Model file for the job. Use its own axes, mm. A direction names the side the tool comes from. Round coordinates to 2 decimals unless told otherwise and drop trailing zeros. Order: outer loops, then holes, each group sorted by start corner. A loop starts at its lowest first (then second) coordinate and runs counter-clockwise, first axis right, second up. Notation, with made-up numbers: (74.5, -23) - (83.5, -23) arc R20 cw to (83.5, -9) - close; hole circle Ø2 at (81.25, 38). An arc over 180 degrees is marked (long way). Answer as CSV lines item,"result". Start each with the question number.
1. Band-saw the part on D-D on z = -4. List the corners of the cut face in (x, y).
2. 3-axis set-ups, long thin cutter, end or side, ignore diameter. For faces 1 (the face through (2, -12, -3)), 2 (the face through (-2, 7, 0)), 3 (the face through (19, 28, 0)): which of +Z, -Z, +X, -X, +Y, -Y reach the whole face in a straight line?
3. Pin check, flat tips, straight feed: pin 1 Ø4 at (x, z) = (2, 1.5) entering from -Y; pin 2 Ø2 at (x, z) = (1, 6) entering from -Y; pin 3 Ø1.5 at (x, z) = (-2, -2.5) entering from +Y; pin 4 Ø1.5 at (x, y) = (2, -13) entering from +Z. Stop position of each tip, or through.
4. Band-saw the part on B-B on y = 24.5. List the corners of the cut face in (x, z).
5. Band-saw the part on C-C on x = 0.75. List the corners of the cut face in (y, z).
6. Band-saw the part on A-A on z = 0. List the corners of the cut face in (x, y), then the cut area to 4 significant figures.
7. Wall check: line 1 along Z through (x, y) = (15.5, 25); line 2 along X through (y, z) = (28, 0.25); line 3 along Y through (x, z) = (2.15, 0). Give the ranges that are in metal, low to high. Write a range as [from, to].
8. Pull direction X, two halves, no side cores. Call faces 4 (the face through (2.46, -4.88, 1.08)), 5 (the face through (19, 8, -14)), 6 (the face through (13, 28, -3)): released by +X, released by -X, zero draft, split by the parting line, or undercut.
```python
from build123d import *

# Parameters (mm, degrees)
SKETCH_1_R          = 5
EXTRUDE_1_DEPTH     = 5
EXTRUDE_2_DEPTH     = 21
FILLET_1_R          = 5
SKETCH_3_W          = 30
SKETCH_3_H          = 27
EXTRUDE_3_DEPTH     = 5
CUT_EXTRUDE_1_DEPTH = 50.037074512


with BuildPart() as part:
    # Sketch 1 → Extrude 1 (new body)
    # profile 1 of 5: a face of its own
    with BuildSketch(Plane(origin=(0, 0, 0), x_dir=(0, 0, -1), z_dir=(1, 0, 0))):
        with BuildLine():
            Line((-15, 30), (15, 30))
            ThreePointArc((15, 30), (0, 45), (-15, 30))
        make_face()
    # profile 2 of 5: a face of its own
    with BuildSketch(Plane(origin=(0, 0, 0), x_dir=(0, 0, -1), z_dir=(1, 0, 0))):
        with BuildLine():
            Line((-15, 45), (-15, 30))
            ThreePointArc((-15, 30), (-10.606601718, 40.606601718), (0, 45))
            Line((0, 45), (-15, 45))
        make_face()
    # profile 3 of 5: a face of its own
    with BuildSketch(Plane(origin=(0, 0, 0), x_dir=(0, 0, -1), z_dir=(1, 0, 0))):
        with BuildLine():
            ThreePointArc((0, 45), (10.606601718, 40.606601718), (15, 30))
            Line((15, 30), (15, 45))
            Line((15, 45), (0, 45))
        make_face()
    # profile 4 of 5: a face of its own
    with BuildSketch(Plane(origin=(0, 0, 0), x_dir=(0, 0, -1), z_dir=(1, 0, 0))):
        with BuildLine():
            Line((-15, 7), (-15, 0))
            ThreePointArc((-15, 0), (-11.618950039, -9.486832981), (-3, -14.696938457))
            Line((-3, -14.696938457), (-3, -8.5))
            Line((-3, -8.5), (3, -8.5))
            Line((3, -8.5), (3, -14.696938457))
            ThreePointArc((3, -14.696938457), (11.618950039, -9.486832981), (15, 0))
            Line((15, 0), (15, 7))
            Line((15, 7), (12, 7))
            Line((12, 7), (12, 27))
            Line((12, 27), (-12, 27))
            Line((-12, 27), (-12, 7))
            Line((-12, 7), (-15, 7))
        make_face()
        Circle(SKETCH_1_R, mode=Mode.SUBTRACT)
    # profile 5 of 5: a face of its own
    with BuildSketch(Plane(origin=(0, 0, 0), x_dir=(0, 0, -1), z_dir=(1, 0, 0))):
        Polygon((-15, 30), (-15, 7), (-12, 7), (-12, 27), (12, 27), (12, 7), (15, 7), (15, 30), align=None)
    extrude(amount=EXTRUDE_1_DEPTH)

    # Sketch 1_4 → Extrude 2 (add)
    with BuildSketch(Plane(origin=(0, 0, 0), x_dir=(0, 0, -1), z_dir=(1, 0, 0))):
        Polygon((-15, 30), (-15, 7), (-12, 7), (-12, 27), (12, 27), (12, 7), (15, 7), (15, 30), align=None)
    extrude(amount=EXTRUDE_2_DEPTH)

    # Fillet 1
    fillet_1_edges = [part.edges().sort_by_distance(p)[0] for p in [
        (21, 7, -13.5),
        (21, 7, 13.5),
    ]]
    fillet(fillet_1_edges, radius=FILLET_1_R)

    # Sketch 3 → Extrude 3 (add)
    with BuildSketch(Plane.ZY):
        with Locations((0, 20.5)):
            Rectangle(SKETCH_3_W, SKETCH_3_H)
    extrude(amount=EXTRUDE_3_DEPTH)

    # Sketch 4 → Cut-Extrude 1 (cut, through all)
    with BuildSketch(Plane.XZ.offset(-27)):
        with BuildLine():
            Line((10, 3), (16, 3))
            ThreePointArc((16, 3), (19, 0), (16, -3))
            Line((16, -3), (10, -3))
            ThreePointArc((10, -3), (7, 0), (10, 3))
        make_face()
    extrude(amount=-CUT_EXTRUDE_1_DEPTH, mode=Mode.SUBTRACT)


solid = part.part
```
Reply:
1,outline,"(-5, 7) - (0, 7) - (0, 3) - (5, 3) - (5, 27) - (21, 27) - (21, 30) - (5, 30) - (5, 45) - (0, 45) - (0, 34) - (-5, 34) - close; (0, -14.46) - (5, -14.46) - (5, -3) - (0, -3) - close"
2,face 1,"+X, -X, -Y"
2,face 2,"+Z, -Z, -X, -Y"
2,face 3,"+Y, -Y"
3,pin 1,"stops at y = -14.7"
3,pin 2,"stops at y = -14.14"
3,pin 3,"stops at y = 34"
3,pin 4,"stops at z = 8.66"
4,outline,"(-5, -15) - (21, -15) - (21, -12) - (5, -12) - (5, 12) - (21, 12) - (21, 15) - (-5, 15) - close"
5,outline,"(-14.7, -3) arc R15 ccw to (0, -15) - (45, -15) - (45, 15) - (0, 15) arc R15 ccw to (-14.7, 3) - (-8.5, 3) - (-8.5, -3) - close; hole circle Ø10 at (0, 0)"
6,outline,"(-5, 7) - (0, 7) - (0, 5) - (5, 5) - (5, 27) - (7, 27) - (7, 30) - (5, 30) - (5, 45) - (0, 45) - (0, 34) - (-5, 34) - close; (0, -8.5) - (5, -8.5) - (5, -5) - (0, -5) - close; (19, 27) - (21, 27) - (21, 30) - (19, 30) - close"
6,area,"364.5 mm2"
7,line 1,"z = [-15, -12], [12, 15]"
7,line 2,"x = [-5, 7.01], [18.99, 21]"
7,line 3,"y = [-8.5, -5], [5, 45]"
8,face 4,"zero draft"
8,face 5,"released by +X"
8,face 6,"undercut"
